from build123d import *

# Parameters (mm, degrees)
SKETCH1_R                = 4.7625
SKETCH1_R_2              = 1.5875
BOSS_EXTRUDE1_DEPTH      = 6.35
M2_5X0_45_TAPPED_HOLE1_D = 2.05
F_1_4_20_TAPPED_HOLE1_D  = 5.1054


with BuildPart() as part:
    # Sketch1 → Boss-Extrude1 (new body)
    with BuildSketch(Plane.XY):
        with BuildLine():
            Line((-25.776330412, 7.096223594), (-5.829565224, 14.900207022))
            ThreePointArc((-5.829565224, 14.900207022), (0, 16), (5.829565224, 14.900207022))
            Line((5.829565224, 14.900207022), (25.776330412, 7.096223594))
            ThreePointArc((25.776330412, 7.096223594), (28.694445061, 5.063367965), (30.372165524, 1.92758271))
            Line((30.372165524, 1.92758271), (50.8, -76.2))
            Line((50.8, -76.2), (-50.8, -76.2))
            Line((-50.8, -76.2), (-30.372165524, 1.92758271))
            ThreePointArc((-30.372165524, 1.92758271), (-28.694445061, 5.063367965), (-25.776330412, 7.096223594))
        make_face()
        Circle(SKETCH1_R, mode=Mode.SUBTRACT)
        with Locations((-31.75, -38.1)):
            Circle(SKETCH1_R_2, mode=Mode.SUBTRACT)
        with Locations((31.75, -38.1)):
            Circle(SKETCH1_R_2, mode=Mode.SUBTRACT)
        with Locations((-31.75, -63.5)):
            Circle(SKETCH1_R_2, mode=Mode.SUBTRACT)
        with Locations((31.75, -63.5)):
            Circle(SKETCH1_R_2, mode=Mode.SUBTRACT)
    extrude(amount=BOSS_EXTRUDE1_DEPTH)

    # M2.5x0.45 Tapped Hole1 (through all)
    with Locations(Plane(origin=(0, 0, 0), x_dir=(-1, 0, 0), z_dir=(0, 0, -1))):
        with Locations((-22.999999974, 0), (22.999999974, 0)):
            Hole(M2_5X0_45_TAPPED_HOLE1_D / 2)

    # 1/4-20 Tapped Hole1 (through all)
    with Locations(Plane.XY.offset(6.35)):
        with Locations((-31.75, -38.1), (-31.75, -63.5), (31.75, -63.5), (31.75, -38.1)):
            Hole(F_1_4_20_TAPPED_HOLE1_D / 2)


solid = part.part
Check sheet for the modelled part. Datum: model origin and axes. Units: mm. Round coordinates to 2 decimals unless told otherwise and drop trailing zeros. Write each loop counter-clockwise with the first axis right and the second up, starting at its lowest first coordinate (ties: lowest second). Pieces come first, ordered by that corner, then holes. Notation, with made-up numbers: (-14, -12) - (6, -12) arc R19 cw to (6, 0) - close; hole circle Ø6 at (-8, 17). An arc over 180 degrees is marked (long way). Return JSON: item names as keys, results as strings.
Q1. Draft check along Y on faces 1 (the flat face through (1, -76.2, 3)), 2 (the cylindrical face through (29.4, -64.5, 3.1)), 3 (the flat face through (-15.943, 10.944, 3.131)). Enter one of: released by +Y, released by -Y, zero draft, split by the parting line, or undercut.
Returned:
{"face 1": "released by -Y", "face 2": "undercut", "face 3": "released by +Y"}
Q2. Depth check by flat-ended pin: P1, Ø6, axis at x = -31.75, y = -63.5, coming from the +Z side; P2, Ø2, axis at x = -24, z = 3, coming from the +Y side. Enter the tip coordinate at first touch or a pass-through.
Returned:
{"P1": "stops at z = 6.35", "P2": "stops at y = 8.18"}
Q3. Scan lines: L1, parallel to X at y = -61.5, z = 1; L2, parallel to X at y = -0.5, z = 5.25; L3, parallel to X at y = -65.5, z = 1.5. Record each from-to range of solid material in increasing order. Write a range as from..to.
Returned:
{"L1": "x = -46.96..-33.34, -30.16..30.16, 33.34..46.96", "L2": "x = -31.01..-23.89, -22.11..-4.74, 4.74..22.11, 23.89..31.01", "L3": "x = -48..-33.34, -30.16..30.16, 33.34..48"}
Q4. Cross-section at D-D (x = 16). Record the boundary of the cut face in (y, z), then the cut area to 3 significant figures.
Returned:
{"outline": "(-76.2, 0) - (10.92, 0) - (10.92, 6.35) - (-76.2, 6.35) - close", "area": "553 mm²"}
Q5. Cross-section at C-C (x = 31.75). Record the boundary of the cut face in (y, z).
Returned:
{"outline": "(-76.2, 0) - (-66.05, 0) - (-66.05, 6.35) - (-76.2, 6.35) - close; (-60.95, 0) - (-40.65, 0) - (-40.65, 6.35) - (-60.95, 6.35) - close; (-35.55, 0) - (-3.34, 0) - (-3.34, 6.35) - (-35.55, 6.35) - close"}
Q6. Cross-section at A-A (z = 1). Give the number of separate pieces and of enclosed holes in the cut face, then the cut area to 3 significant figures.
Returned:
{"separate pieces": "1", "enclosed holes": "7", "area": "6,740 mm²"}
Q7. Cross-section at B-B (y = -38.1). Record the boundary of the cut face in (x, z).
Returned:
{"outline": "(-40.84, 0) - (-34.3, 0) - (-34.3, 6.35) - (-40.84, 6.35) - close; (-29.2, 0) - (29.2, 0) - (29.2, 6.35) - (-29.2, 6.35) - close; (34.3, 0) - (40.84, 0) - (40.84, 6.35) - (34.3, 6.35) - close"}
